```python
from build123d import *

# Parameters (mm, degrees)
F0_R     = 2.5
F1_DEPTH = 6
F2_R     = 5
F3_DEPTH = 10
F4_R     = 3.5
F5_DEPTH = 5.1
F6_R     = 5
F7_DEPTH = 5
F8_SIZE  = 0.5
F9_R     = 4.99999


# Not quite as in the source:
# - a fillet or chamfer is up to 0.001 mm smaller than in the source, because OpenCascade refuses the exact size


with BuildPart() as f1:
    # F0 (on Top) → F1 (new body)
    with BuildSketch(Plane.XY):
        Circle(F0_R)
    extrude(amount=F1_DEPTH)

    # F2 (on face) → F3 (join)
    with BuildSketch(Plane.XY.offset(6)):
        Circle(F2_R)
    extrude(amount=F3_DEPTH)

    # F4 (on face) → F5 (join)
    with BuildSketch(Plane.XY.offset(16)):
        Circle(F4_R)
    extrude(amount=F5_DEPTH)

    # F6 (on face) → F7 (join)
    with BuildSketch(Plane.XY.offset(21.1)):
        Circle(F6_R)
    extrude(amount=F7_DEPTH)

    # F8
    f8_edges = [f1.edges().sort_by_distance(p)[0] for p in [
        (-2.5, 0, 0),
    ]]
    chamfer(f8_edges, length=F8_SIZE)

    # F9 (radius 5 in the source; OpenCascade refuses exactly that, so slightly less here)
    f9_edges = [f1.edges().sort_by_distance(p)[0] for p in [
        (-5, 0, 26.1),
    ]]
    fillet(f9_edges, radius=F9_R)


solid = f1.part
```
Source: CAD feature listing. Evaluate the final solid. Frame: model axes, mm. A direction names the side the tool comes from. Coordinates: 2 decimals unless noted, no trailing zeros. Loops run counter-clockwise (first coordinate to the right, second up) from the corner with the lowest first, then second, coordinate; pieces in that order, holes last. Notation, with made-up numbers: M 75.25,-9.5 L 87.25,-9.5 A15 ccw 87.25,2.5 Z; hole C 71.25,83.25 d11. An arc over 180 degrees is marked long. Put each result on its own line as item: value. Start each with the question number.
1) Reachability of faces 5 (the face through (-1.08, -4.88, 10.93)), 6 (the face through (2.2, -3.3, 21.1)) from +Z, -Z, +X, -X, +Y, -Y: full face, straight path, thin tool, end or side. Return the list, or none.
2) Cut plane A-A on z = 15. Return the cut outline in (x, y), then the cut area to 3 significant figures.
3) Contact query for flat-ended pins moving along their axis: pin 1 Ø1.5 at (x, y) = (-2.5, -1.5) entering from -Z; pin 2 Ø6 at (y, z) = (-3.5, 8.5) entering from +X; pin 3 Ø4 at (x, z) = (2.5, 19) entering from -Y. Output: stop coordinate, or through.
4) Cut plane B-B on z = 19.5. Return the cut outline in (x, y).
5) Ray query, L1, parallel to X at y = 1.5, z = 5.75; L2, parallel to Z at x = -4, y = 1.5; L3, parallel to X at y = 1.25, z = 22.5. Return the intervals inside material, ascending. Write a range as from..to.
6) Pull-direction query (Z, two-part tool) for faces 1 (the face through (2.2, -3.3, 16)), 2 (the face through (2, -2, 6)), 3 (the face through (-0.54, -2.44, 3.21)), 4 (the face through (3.233, -1.341, 18.514)); classes: pulls with the +Z half, pulls with the -Z half, needs draft (parallel to the pull), parting line crosses it, or undercut.
The answers:
1. face 5: +Z, -Z
1. face 6: none
2. outline: C 0,0 d10
2. area: 78.5 mm²
3. pin 1: stops at z = 0.17
3. pin 2: stops at x = 4.97
3. pin 3: stops at y = -3.46
4. outline: C 0,0 d7
5. L1: x = -2..2
5. L2: z = 6..16, 21.1..23.7
5. L3: x = -4.63..4.63
6. face 1: undercut
6. face 2: pulls with the -Z half
6. face 3: needs draft
6. face 4: undercut
